The drawing under review shows one solid part. Ordinate dimensions are in mm from its lowest x, y, z. A direction names the side the tool comes from. Give positions to 0.01 mm unless a question says otherwise; leave off trailing zeros. Order: outer loops, then holes, each group sorted by start corner. A loop starts at its lowest first (then second) coordinate and runs counter-clockwise, first axis right, second up. Notation, with made-up numbers: (6, -13.5) - (37, -13.5) arc R26 ccw to (37, 1.5) - close; hole circle Ø3 at (-8.75, 35). An arc over 180 degrees is marked (long way). Use CSV: the item, a comma, the result in double quotes.
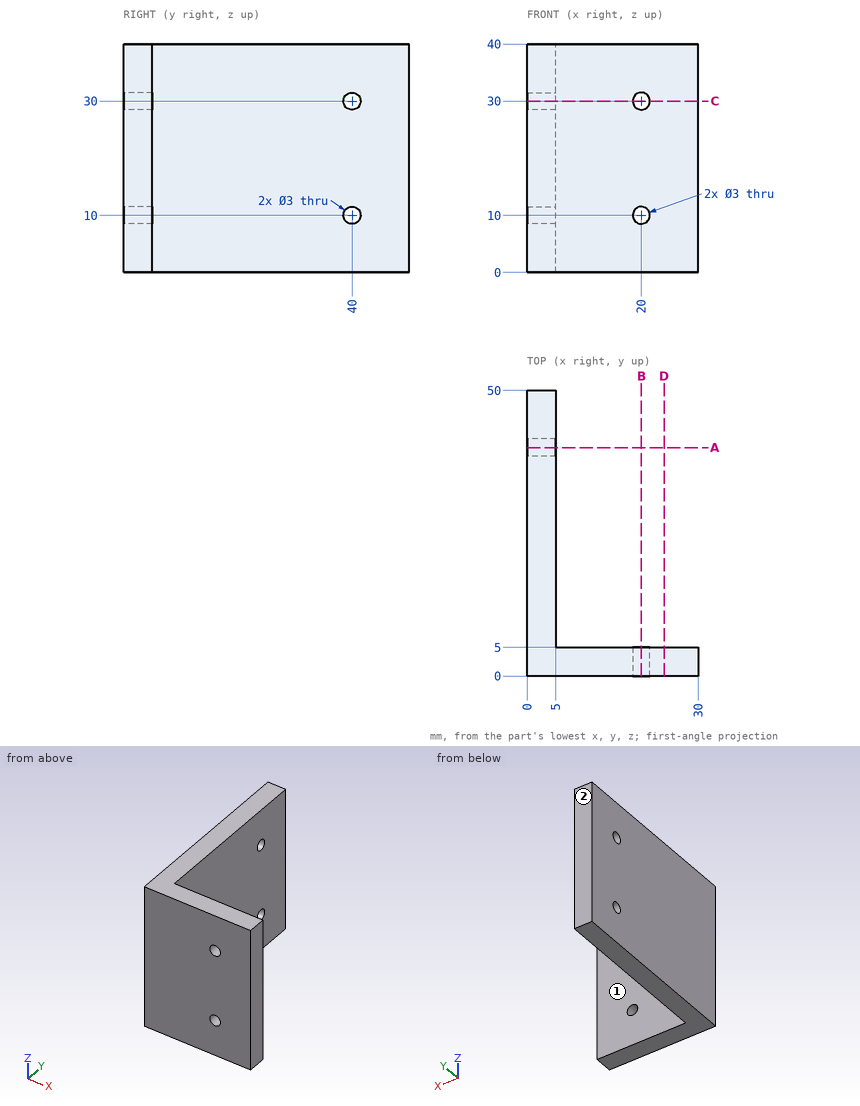
Item 1: Take a section at D-D, the plane x = 24. Give the boundary of the cut face in (y, z).
Results list:
outline,"(0, 0) - (5, 0) - (5, 40) - (0, 40) - close"
Item 2: Wall thickness on L1, parallel to Z at x = 20, y = 1.6; L2, parallel to X at y = 6.5, z = 11: over which ranges is each line inside the solid? List them lowest first.
Results list:
L1,"z = 0 to 8.5, 11.5 to 28.5, 31.5 to 40"
L2,"x = 0 to 5"
Item 3: Clearance check with flat-ended pins moving along their axes: pin 1 (8 mm diameter, centred on x = 5.5, z = 16, fed in from +Y); pin 2 (20 mm diameter, centred on y = 35, z = 29.5, fed in from +X); pin 3 (1.5 mm diameter, centred on x = 11.5, z = 23, fed in from +Y). State where each tip first meets the part, or that it passes through.
Results list:
pin 1,"stops at y = 50"
pin 2,"stops at x = 5"
pin 3,"stops at y = 5"
Item 4: Tool access review of the marked faces 1 and 2: name each direction out of +Z, -Z, +X, -X, +Y, -Y from which nothing blocks a thin tool from reaching the whole face with its end or side.
Results list:
face 1,"+Z, -Z, +X, +Y"
face 2,"+Z, -Z, +X, -X, +Y"
Item 5: Take a section at A-A, the plane y = 40. Give the boundary of the cut face in (x, z).
Results list:
outline,"(0, 0) - (5, 0) - (5, 8.5) - (0, 8.5) - close; (0, 11.5) - (5, 11.5) - (5, 28.5) - (0, 28.5) - close; (0, 31.5) - (5, 31.5) - (5, 40) - (0, 40) - close"
Item 6: Take a section at C-C, the plane z = 30. Give the boundary of the cut face in (x, y).
Results list:
outline,"(0, 0) - (18.5, 0) - (18.5, 5) - (5, 5) - (5, 38.5) - (0, 38.5) - close; (0, 41.5) - (5, 41.5) - (5, 50) - (0, 50) - close; (21.5, 0) - (30, 0) - (30, 5) - (21.5, 5) - close"
